Autodesk Inventor part; units mm, degrees
ref_plane "YZ Plane" through (0, 0, 0) normal (1, 0, 0) x (0, 1, 0)
ref_plane "XZ Plane" through (0, 0, 0) normal (0, 1, 0) x (-1, 0, 0)
ref_plane "XY Plane" through (0, 0, 0) normal (0, 0, 1) x (1, 0, 0)
sketch "Sketch1" plane through (0, 0, 0) normal (1, 0, 0) x (0, 1, 0)
  line L0 (0, 0) -> (1.25, 0)
  line L1 (1.25, 0) -> (1.25, -25.25)
  line L2 (1.25, -25.25) -> (0, -25.25)
  line L3 (0, -25.25) -> (0, 0)
  line L4 (4.625, -1.625) -> (0.625, 0.3009)
  line L5 (0.625, 0.3009) -> (-3.375, -1.625)
  line L6 (-3.375, -23.625) -> (0.625, -25.5509)
  line L7 (0.625, -25.5509) -> (4.625, -23.625)
  line L8 (4.625, 2.3009) -> (-3.375, 2.3009)
  line L9 (-3.375, 2.3009) -> (-3.375, -27.5509)
  line L10 (-3.375, -27.5509) -> (4.625, -27.5509)
  line L11 (4.625, -27.5509) -> (4.625, 2.3009)
  line L12 (-3.375, 2.3009) -> (-5.375, 2.3009)
  line L13 (-5.375, 2.3009) -> (-5.375, -27.5509)
  line L14 (-5.375, -27.5509) -> (-3.375, -27.5509)
  line L15 (-3.375, -27.5509) -> (-3.375, 2.3009)
  line L16 (-1.0385, -0.5) -> (2.2885, -0.5)
  line L17 (-1.0385, -24.75) -> (2.2885, -24.75)
  point P0 (0, -24.75)
  point P1 (0, -0.5)
  point P2 (1.25, -0.5)
  point P3 (1.25, -24.75)
  dimension "d0" = 1.25
  dimension "d1" = 25.25
  dimension "d2" = 0.625
  dimension "d3" = 2
  dimension "d4" = 2
  dimension "d5" = 8
  dimension "d6" = 22
  dimension "d7" = 2
  dimension "d8" = 0.5
  dimension "d9" = 0.5
extrude "Extrusion1" add sketch "Sketch1" along normal blind 25 contours L5 L4 L0 | L5 L9 L8 L11 L4 | L3 L16 L5 | L4 L16 L1 | L3 L6 L17 | L9 L14 L13 L12 | L17 L7 L1 | L6 L7 L11 L10 L9 | L2 L7 L6
equation "\"d2\" = 0.5 * d0"
properties part number "RaspberryPi Camera Slotted Mount"
CAD build for the part. Positions are in the model's coordinates, mm. A direction names the side the tool comes from. Coordinates: 2 decimals unless noted, no trailing zeros. Order: outer loops, then holes, each group sorted by start corner. A loop starts at its lowest first (then second) coordinate and runs counter-clockwise, first axis right, second up.
(1) Mould opens along Y. For faces 4 (the face through (12, 0, 2.301)), 5 (the face through (12.3, -0.5, -24.75)), 6 (the face through (12, 4.625, 0)) say: released by +Y, released by -Y, zero draft, split by the parting line, or undercut.
Solution:
face 4: zero draft
face 5: undercut
face 6: released by +Y
(2) Which spindle directions (+Z, -Z, +X, -X, +Y, -Y) get a long thin tool onto all of the face, cutting with end or side? Do faces 1 (the face through (25, -4, -12)), 2 (the face through (12, -3.375, -12)), 3 (the face through (12, 1, -25.25)). Say none if no direction does.
Solution:
face 1: +Z, -Z, +X, +Y, -Y
face 2: +X, -X, +Y
face 3: +X, -X
(3) Saw through at D-D, the plane y = -1.5. Write the cut outline in (x, z), and give its area (3 significant figures).
Solution:
outline: (0, -27.55) - (25, -27.55) - (25, -24.53) - (0, -24.53) - close; (0, -0.72) - (25, -0.72) - (25, 2.3) - (0, 2.3) - close
area: 151 mm2
(4) Pin check, flat tip, straight feed: pin 1 Ø10 at (x, z) = (19, -12) entering from +Y (3 decimals). Stop position of the tip, or through.
Solution:
pin 1: stops at y = -3.375
(5) Drill centre lines: L1, parallel to Z at x = 20.5, y = 2.25; L2, parallel to Z at x = 16.5, y = 1; L3, parallel to Y at x = 22.75, z = -11.25 (3 decimals). Where is each one in solid material? Low to high.
Solution:
L1: z = -27.55 to -24.75, -0.5 to 2.3
L2: z = -27.55 to -25.25, 0 to 2.3
L3: y = -5.375 to -3.375
(6) Saw through at A-A, the plane y = 4. Write the cut outline in (x, z).
Solution:
outline: (0, -27.55) - (25, -27.55) - (25, -23.93) - (0, -23.93) - close; (0, -1.32) - (25, -1.32) - (25, 2.3) - (0, 2.3) - close
(7) Saw through at B-B, the plane z = -13. Write the cut outline in (x, y) (3 decimals).
Solution:
outline: (0, -5.375) - (25, -5.375) - (25, -3.375) - (0, -3.375) - close
